Design review of the part built by this model. Coordinates are the model's own, in mm. Round coordinates to 2 decimals unless told otherwise and drop trailing zeros. Write item = value, one per line.
from build123d import *

# Parameters (mm, degrees)
EXTRUDE_1_DEPTH       = 350
EXTRUDE_3_DEPTH       = 350
PATTERN_CURVE_1_COUNT = 11
PATTERN_CURVE_1_PITCH = 10
SKETCH_3_R            = 2.25
CUT_EXTRUDE_1_DEPTH   = 6
SKETCH_4_R            = 2.25
SKETCH_4_R_2          = 1.6
CUT_EXTRUDE_2_DEPTH   = 6


with BuildPart() as part:
    # Эскиз1 → Вытянуть1 (new body)
    with BuildSketch(Plane.XY):
        with BuildLine():
            Line((0, 40), (1.528979332, 40))
            ThreePointArc((1.528979332, 40), (2.225614441, 39.717425624), (2.528547087, 39.029399052))
            Line((2.528547087, 39.029399052), (3.5, 6))
            Line((3.5, 6), (118.5, 6))
            Line((118.5, 6), (119.471452913, 39.029399052))
            ThreePointArc((119.471452913, 39.029399052), (119.774385559, 39.717425624), (120.471020668, 40))
            Line((120.471020668, 40), (122, 40))
            Line((122, 40), (122, 0))
            Line((122, 0), (0, 0))
            Line((0, 0), (0, 40))
        make_face()
    extrude(amount=EXTRUDE_1_DEPTH)

    # Эскиз2 → Вытянуть3 (add)
    with BuildSketch(Plane.XY.offset(350)):
        with BuildLine():
            Line((10.5, 39.5), (9.25, 6))
            Line((9.25, 6), (12.75, 6))
            Line((12.75, 6), (11.5, 39.5))
            ThreePointArc((11.5, 39.5), (11, 40), (10.5, 39.5))
        make_face()
    extrude_3 = extrude(amount=-EXTRUDE_3_DEPTH)

    # Кривая1: Вытянуть3 ×11
    with Locations(*[(i * PATTERN_CURVE_1_PITCH, 0, 0) for i in range(1, PATTERN_CURVE_1_COUNT)]):
        add(extrude_3)

    # Эскиз3 → Вырез-Вытянуть1 (cut)
    with BuildSketch(Plane.XZ):
        with Locations((26, 342)):
            Circle(SKETCH_3_R)
        with Locations((96, 342)):
            Circle(SKETCH_3_R)
        with Locations(Location((96, 8, 0), (0, 0, 180))):
            Circle(SKETCH_3_R)
        with Locations(Location((26, 8, 0), (0, 0, 180))):
            Circle(SKETCH_3_R)
    extrude(amount=-CUT_EXTRUDE_1_DEPTH, mode=Mode.SUBTRACT)

    # Эскиз4 → Вырез-Вытянуть2 (cut)
    with BuildSketch(Plane.XZ):
        with Locations((12.5, 40)):
            Circle(SKETCH_4_R)
        with Locations((12.5, 92)):
            Circle(SKETCH_4_R)
        with Locations((32, 25)):
            Circle(SKETCH_4_R_2)
        with Locations((80, 25)):
            Circle(SKETCH_4_R_2)
        with Locations((80, 91)):
            Circle(SKETCH_4_R_2)
        with Locations((32, 91)):
            Circle(SKETCH_4_R_2)
        with Locations((37.5, 115)):
            Circle(SKETCH_4_R_2)
        with Locations((37.5, 255)):
            Circle(SKETCH_4_R_2)
        with Locations((72, 128)):
            Circle(SKETCH_4_R_2)
        with Locations((72, 195)):
            Circle(SKETCH_4_R_2)
        with Locations((26, 295)):
            Circle(SKETCH_4_R)
        with Locations((26, 320)):
            Circle(SKETCH_4_R)
    extrude(amount=-CUT_EXTRUDE_2_DEPTH, mode=Mode.SUBTRACT)


solid = part.part
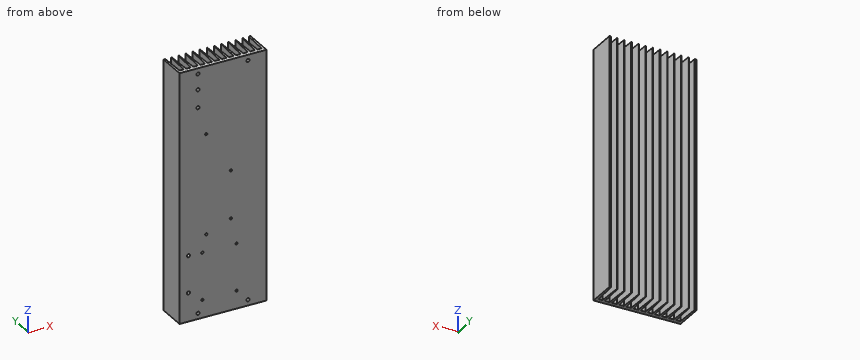
1) Clearance check with flat-ended pins moving along their axes: pin 1 Ø3 at (x, z) = (32, 91) entering from -Y; pin 2 Ø2 at (x, z) = (85, 234) entering from +Y; pin 3 Ø1 at (x, y) = (87.5, 9.5) entering from +Z. State where each tip first meets the part, or that it passes through.
Findings:
pin_1 = 6
pin_2 = 6
pin_3 = through
2) We need section A-A on y = 30.5. Give the number of separate pieces and of enclosed holes in the cut face, and give its area (3 significant figures).
Findings:
separate_pieces = 13
enclosed_holes = 0
area = 8,380 mm^2
3) To check wall thickness, follow L1, parallel to Z at x = 12.5, y = 2.4; L2, parallel to Z at x = 26, y = 3.1; L3, parallel to X at y = 2, z = 25. State the ranges of each line that lie inside material, in increasing order. Write a range as from..to.
Findings:
L1 = 0..37.75, 42.25..89.75, 94.25..350
L2 = 0..5.75, 10.25..292.75, 297.25..317.75, 322.25..339.75, 344.25..350
L3 = 0..30.4, 33.6..78.4, 81.6..122
